Autodesk Inventor part; units mm, degrees
ref_plane "YZ Plane" through (0, 0, 0) normal (1, 0, 0) x (0, 1, 0)
ref_plane "XZ Plane" through (0, 0, 0) normal (0, 1, 0) x (-1, 0, 0)
ref_plane "XY Plane" through (0, 0, 0) normal (0, 0, 1) x (1, 0, 0)
sketch "Sketch1" plane through (0, 0, 0) normal (0, 1, 0) x (-1, 0, 0)
  arc A0 (-16, 0) -> (-15.7162, 3) centre (0, 0) ccw
  arc A1 (-11.6822, -17.4507) -> (-14.7951, 14.9032) centre (0, 0) ccw
  line L0 (-16, 0) -> (-184, 0)
  line L1 (-184, 0) -> (-184, -9)
  line L2 (-184, -9) -> (-39.4968, -9)
  arc A2 (-11.6822, -17.4507) -> (-39.4968, -9) centre (-39.4968, -59) ccw
  line L3 (-39, 12) -> (-39, 3)
  line L4 (0, 0) -> (0, 3)
  line L5 (-15.7162, 3) -> (-39, 3)
  line L6 (-39, 3) -> (-39, 12)
  line L7 (-39, 12) -> (-21.8403, 12)
  arc A3 (-21.8403, 12) -> (-14.7951, 14.9032) centre (-21.8403, 22) ccw
  point P0 (-18.9737, -9)
  point P1 (-17.2337, 12)
  dimension "d0" = 32
  dimension "d1" = 42
  dimension "d2" = 168
  dimension "d3" = 9
  dimension "d4" = 50
  dimension "d7" = 3
  dimension "d8" = 39
  dimension "d9" = 9
  dimension "d10" = 3
  dimension "d11" = 39
  dimension "d12" = 10
extrude "Extrusion1" add sketch "Sketch1" along normal blind 50
hole "Hole1" at (32, 10, 12) direction (0, 0, -1) diameter 5.5 end through all counterbore diameter 10 counterbore depth 4
hole "Hole2" at (32, 40, 12) direction (0, 0, -1) diameter 5.5 end through all counterbore diameter 10 counterbore depth 4
sketch "Sketch3" plane through (16, 0, 0) normal (0, 0, 1) x (1, 0, 0)
  point P0 (-16, 0)
fillet "Fillet1" radius 2.5 2 edges at (39, 25, 12) (39, 25, 3)
sketch "Sketch4" plane through (0, 0, 0) normal (0, 1, 0) x (-1, 0, 0)
  point P0 (0, 0)
sketch "Sketch5" plane through (0, 0, 0) normal (0, 0, 1) x (1, 0, 0)
  line L0 (0, 0) -> (0, 17)
  line L1 (14.7951, 50) -> (-21, 50)
  line L2 (-8, 17) -> (-40, 17)
  line L3 (-40, 17) -> (-40, 33)
  line L4 (-40, 33) -> (-8, 33)
  line L5 (0, 25) -> (0, 25)
  arc A0 (0, 25) -> (-8, 33) centre (-8, 25) ccw
  arc A1 (-8, 17) -> (0, 25) centre (-8, 25) ccw
  point P0 (11.6822, 50)
  point P1 (0, 33)
  dimension "d41" = 17
  dimension "d42" = 40
  dimension "d43" = 16
  dimension "d44" = 40
  dimension "d45" = 8
extrude "Extrusion3" cut sketch "Sketch5" along normal through all both and the other way through all
sketch "Sketch8" plane through (16, 0, 0) normal (0, 0, 1) x (1, 0, 0)
  line L0 (-16, 0) -> (-16, 50)
  line L1 (-32, 50) -> (0, 50)
  line L2 (-16, 50) -> (34, 50)
  line L3 (0, 50) -> (168, 50)
  line L4 (34, 50) -> (34, 33)
  line L5 (34, 33) -> (154, 33)
  line L6 (168, 0) -> (168, 50)
  line L7 (51.1, 0) -> (173.3862, 0) construction
  line L8 (34, 50) -> (38, 50)
  line L9 (38, 50) -> (38, 41.5)
  circle A0 centre (38, 41.5) radius 3.1
  circle A1 centre (48, 41.5) radius 3.1
  circle A2 centre (58, 41.5) radius 3.1
  circle A3 centre (68, 41.5) radius 3.1
  circle A4 centre (78, 41.5) radius 3.1
  circle A5 centre (88, 41.5) radius 3.1
  circle A6 centre (98, 41.5) radius 3.1
  circle A7 centre (108, 41.5) radius 3.1
  circle A8 centre (118, 41.5) radius 3.1
  circle A9 centre (128, 41.5) radius 3.1
  circle A10 centre (138, 41.5) radius 3.1
  circle A11 centre (148, 41.5) radius 3.1
  circle A12 centre (158, 41.5) radius 3.1
  arc A13 (34, 9.0247) -> (154, 33) centre (32.6984, 327.8368) ccw
  line L10 (34, 0) -> (168, 0)
  line L11 (168, 0) -> (168, 33)
  arc A14 (34, 0) -> (51.1, 0) centre (42.55, 253.8424) ccw
  line L12 (34, 9.0247) -> (34, 33)
  arc A15 (34, 0) -> (168, 33) centre (42.55, 253.8424) ccw
  point P0 (-0.2838, 50)
  dimension "d49" = 50
  dimension "d50" = 17
  dimension "d54" = 4
  dimension "d55" = 8.5
  dimension "d56" = 6.2
  dimension "d59" = 10
  dimension "d73" = 120
  dimension "d74" = 23.9753
extrude "Extrusion4" cut sketch "Sketch8" against normal through all contours L6 L10 A15 | A0 | L5 A13 L12 | A1 | A2 | A3 | A4 | A5 | A6 | A7 | A8 | A9 | A10 | A11 | A12
fillet "Fillet2" radius 4 1 edges at (170, 33, -4.5)
fillet "Fillet3" radius 4 2 edges at (50, 33, -4.5) (50, 9.0247, -4.5)
fillet "Fillet4" radius 8 2 edges at (184, 50, -4.5) (184, 33, -4.5)
properties part number "suporte-rodas-esq" material "Aluminium AW-7020"
Verification items for the finished model (mm, model axes). A direction names the side the tool comes from. Round coordinates to 2 decimals unless told otherwise and drop trailing zeros. Write each loop counter-clockwise with the first axis right and the second up, starting at its lowest first coordinate (ties: lowest second). Pieces come first, ordered by that corner, then holes.
1. Gauge pin test, flat ends, axial feed: P1, Ø10, axis at x = 154, y = 41.5, coming from the -Z side; P2, Ø3.5, axis at x = 74, y = 41.5, coming from the -Z side; P3, Ø8, axis at y = 26, z = 5.5, coming from the +X side; P4, Ø5, axis at y = 25.5, z = -9, coming from the -X side. Record the tip position at first contact, or that the pin passes through.
2. Section check D-D on x = 32. State how many separate pieces and enclosed holes the cut face has, plus the area to 3 significant figures.
3. Section check C-C on y = 19. Enter the section's corners in (x, z).
4. Access from +Z, -Z, +X, -X, +Y, -Y to the whole of each face (thin tool, end or side, straight path). Record for faces 4 (the cylindrical face through (101.47, 13.42, -4.44)), 5 (the flat face through (39, 25, 8)), 6 (the flat face through (97, 36, -9)), 7 (the flat face through (34.2, 7.8, 8)).
5. Draft check along Y on faces 1 (the flat face through (80, 36, 0)), 2 (the flat face through (100, 33, -4)), 3 (the flat face through (20, 0, 3.2)). Enter one of: +Y half, -Y half, draft (parallel to the pull), parting line (faces both ways), or undercut.
6. Scan lines: L1, parallel to Y at x = 32, z = 10.25; L2, parallel to Y at x = 32, z = -5.5; L3, parallel to X at y = 40, z = 8.95. Record each from-to range of solid material in increasing order.
7. Section check B-B on x = 124. Enter the section's corners in (y, z).
8. Section check A-A on x = 154. Enter the section's corners in (y, z).
Answer:
1. P1: stops at z = -9
1. P2: passes through
1. P3: stops at x = 39
1. P4: stops at x = 11.12
2. separate pieces: 6
2. enclosed holes: 0
2. area: 688 mm2
3. outline: (-2.71, -20.82) arc R21 ccw to (11.68, -17.45) arc R50 cw to (39.5, -9) - (50, -9) - (50, 0) - (16, 0) arc R16 cw to (-2.71, -15.77) - close; (-2.71, 15.77) arc R16 cw to (15.72, 3) - (36.5, 3) arc R2.5 ccw to (39, 5.5) - (39, 9.5) arc R2.5 ccw to (36.5, 12) - (21.84, 12) arc R10 cw to (14.8, 14.9) arc R21 ccw to (-2.71, 20.82) - close; (127.84, -9) - (155.29, -9) - (155.29, 0) - (127.84, 0) - close
4. face 4: +Z, -Z
4. face 5: +Z, +X, +Y, -Y
4. face 6: -Z, +X, +Y, -Y
4. face 7: +Z
5. face 1: draft
5. face 2: undercut
5. face 3: -Y half
6. L1: y = 0 to 5, 15 to 35, 45 to 50
6. L2: y = 0 to 7.25, 12.75 to 37.25, 42.75 to 50
6. L3: x = -19 to -13.26, 13.26 to 27, 37 to 39
7. outline: (8.43, -9) - (18.04, -9) - (18.04, 0) - (8.43, 0) - close; (33, -9) - (38.4, -9) - (38.4, 0) - (33, 0) - close; (44.6, -9) - (50, -9) - (50, 0) - (44.6, 0) - close
8. outline: (18.47, -9) - (38.4, -9) - (38.4, 0) - (18.47, 0) - close; (44.6, -9) - (50, -9) - (50, 0) - (44.6, 0) - close
